For this review, take the finished solid that the model builds, in its own axes (mm). Face numbers are marked on the shaded views. A direction names the side the tool comes from. Coordinates: 2 decimals unless noted, no trailing zeros. Loops run counter-clockwise (first coordinate to the right, second up) from the corner with the lowest first, then second, coordinate; pieces in that order, holes last. Notation, with made-up numbers: (-11, -19) -> (29, -19) arc R23 cw to (29, 20) -> close; hole circle Ø11 at (-5.75, -32.75). An arc over 180 degrees is marked (long way). Answer in a Markdown table with one row per item.
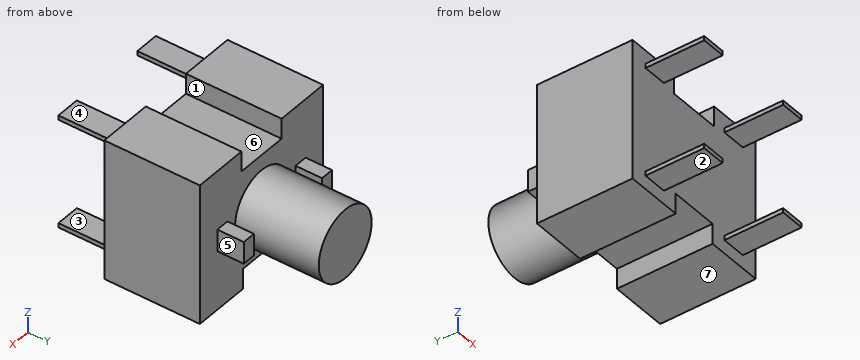
from build123d import *

# Parameters (mm, degrees)
SKETCH1_W           = 18.4
SKETCH1_H           = 15.96
BOSS_EXTRUDE1_DEPTH = 10.85
SKETCH2_W           = 2.75
SKETCH2_H           = 0.5
BOSS_EXTRUDE2_DEPTH = 6.67
SKETCH3_W           = 5.5
SKETCH3_H           = 2.3
SKETCH3_W_2         = 6
CUT_EXTRUDE1_DEPTH  = 18.52
SKETCH4_R           = 3.95
BOSS_EXTRUDE3_DEPTH = 9.5
SKETCH5_W           = 1.5
SKETCH5_H           = 2.5
BOSS_EXTRUDE4_DEPTH = 3


with BuildPart() as part:
    # Sketch1 → Boss-Extrude1 (new body)
    with BuildSketch(Plane(origin=(0, 0, 0), x_dir=(1, 0, 0), z_dir=(0, 1, 0))):
        Rectangle(SKETCH1_W, SKETCH1_H)
    extrude(amount=BOSS_EXTRUDE1_DEPTH)

    # Sketch2 → Boss-Extrude2 (add)
    with BuildSketch(Plane.XZ):
        with Locations((-5.895, -6.2)):
            Rectangle(SKETCH2_W, SKETCH2_H)
        with Locations((-5.895, 6.2)):
            Rectangle(SKETCH2_W, SKETCH2_H)
        with Locations((5.895, -6.2)):
            Rectangle(SKETCH2_W, SKETCH2_H)
        with Locations((5.895, 6.2)):
            Rectangle(SKETCH2_W, SKETCH2_H)
    extrude(amount=BOSS_EXTRUDE2_DEPTH)

    # Sketch3 → Cut-Extrude1 (cut, through all)
    with BuildSketch(Plane(origin=(0, 10.85, 0), x_dir=(1, 0, 0), z_dir=(0, 1, 0))):
        with Locations((0, 6.83)):
            Rectangle(SKETCH3_W, SKETCH3_H)
        with Locations((0, -6.83)):
            Rectangle(SKETCH3_W_2, SKETCH3_H)
    extrude(amount=-CUT_EXTRUDE1_DEPTH, mode=Mode.SUBTRACT)

    # Sketch4 → Boss-Extrude3 (add)
    with BuildSketch(Plane(origin=(0, 10.85, 0), x_dir=(1, 0, 0), z_dir=(0, 1, 0))):
        Circle(SKETCH4_R)
    extrude(amount=BOSS_EXTRUDE3_DEPTH)

    # Sketch5 → Boss-Extrude4 (add)
    with BuildSketch(Plane(origin=(0, 10.85, 0), x_dir=(1, 0, 0), z_dir=(0, 1, 0))):
        with Locations((-5.84, 0)):
            Rectangle(SKETCH5_W, SKETCH5_H)
        with Locations((5.84, 0)):
            Rectangle(SKETCH5_W, SKETCH5_H)
    extrude(amount=BOSS_EXTRUDE4_DEPTH)


solid = part.part
Item 1: For L1, parallel to Z at x = 6.25, y = -1.5; L2, parallel to Y at x = 4.75, z = -4.75; L3, parallel to Y at x = 3, z = 1.5, list the stretches that pass through material, from the lowest coordinate up.
Worked answers:
| item | result |
|---|---|
| L1 | -6.45 to -5.95, 5.95 to 6.45 |
| L2 | 0 to 10.85 |
| L3 | 0 to 20.35 |
Item 2: Take a section at A-A, the plane y = 12.5. State the section outline as (x, z) points, and give its area (3 significant figures).
Worked answers:
| item | result |
|---|---|
| outline | (-6.59, -1.25) -> (-5.09, -1.25) -> (-5.09, 1.25) -> (-6.59, 1.25) -> close; circle Ø7.9 at (0, 0); (5.09, -1.25) -> (6.59, -1.25) -> (6.59, 1.25) -> (5.09, 1.25) -> close |
| area | 56.5 mm² |
Item 3: The part is to be moulded in two halves that separate along X. For the marked faces 5, 6 and 7, say which applies: +X half, -X half, draft (parallel to the pull), parting line (faces both ways), or undercut.
Worked answers:
| item | result |
|---|---|
| face 5 | +X half |
| face 6 | undercut |
| face 7 | draft |
Item 4: For the marked faces 1, 2, 3 and 4, list the 3-axis set-ups (+Z, -Z, +X, -X, +Y, -Y) from which the entire face can be reached by the end or side of a thin tool; tool diameter is ignored.
Worked answers:
| item | result |
|---|---|
| face 1 | +Z, +Y, -Y |
| face 2 | -Z, +X, -X, -Y |
| face 3 | +X, -X, -Y |
| face 4 | +Z, +X, -X, -Y |
Item 5: Take a section at C-C, the plane y = 1.5. State the section outline as (x, z) points.
Worked answers:
| item | result |
|---|---|
| outline | (-9.2, -7.98) -> (-2.75, -7.98) -> (-2.75, -5.68) -> (2.75, -5.68) -> (2.75, -7.98) -> (9.2, -7.98) -> (9.2, 7.98) -> (3, 7.98) -> (3, 5.68) -> (-3, 5.68) -> (-3, 7.98) -> (-9.2, 7.98) -> close |
Item 6: Take a section at D-D, the plane z = 0. State the section outline as (x, y) points, and give its area (3 significant figures).
Worked answers:
| item | result |
|---|---|
| outline | (-9.2, 0) -> (9.2, 0) -> (9.2, 10.85) -> (6.59, 10.85) -> (6.59, 13.85) -> (5.09, 13.85) -> (5.09, 10.85) -> (3.95, 10.85) -> (3.95, 20.35) -> (-3.95, 20.35) -> (-3.95, 10.85) -> (-5.09, 10.85) -> (-5.09, 13.85) -> (-6.59, 13.85) -> (-6.59, 10.85) -> (-9.2, 10.85) -> close |
| area | 284 mm² |
Item 7: Insertion check: pin 1 (0.6 mm diameter, centred on y = -4, z = 6.5, fed in from -X); pin 2 (1.4 mm diameter, centred on x = -6, y = -2, fed in from -Z); pin 3 (0.8 mm diameter, centred on x = 6, y = -4, fed in from +Z); pin 4 (4 mm diameter, centred on y = -1.5, z = -6, fed in from +X). Each pin has a flat end and moves straight along its axis. Give the tip position at first contact, or say it passes through.
Worked answers:
| item | result |
|---|---|
| pin 1 | x = -7.27 |
| pin 2 | z = -6.45 |
| pin 3 | z = 6.45 |
| pin 4 | x = 9.2 |
Item 8: Take a section at B-B, the plane x = 0. State the section outline as (y, z) points.
Worked answers:
| item | result |
|---|---|
| outline | (0, -5.68) -> (10.85, -5.68) -> (10.85, -3.95) -> (20.35, -3.95) -> (20.35, 3.95) -> (10.85, 3.95) -> (10.85, 5.68) -> (0, 5.68) -> close |
